```python
from build123d import *

# Parameters (mm, degrees)
ESQUISSE1_R             = 34.9
BOSS_EXTRU_1_DEPTH      = 4
ESQUISSE4_W             = 3
ESQUISSE4_H             = 15
BOSS_EXTRU_3_DEPTH      = 20
ENL_V_MAT_EXTRU_2_DEPTH = 57.306038753
CONG_1_R                = 5
ESQUISSE6_R             = 2.5
ENL_V_MAT_EXTRU_3_DEPTH = 55.995032503
BOSS_EXTRU_4_DEPTH      = 2
CONG_2_R                = 2


with BuildPart() as part:
    # Esquisse1 → Boss.-Extru.1 (new body)
    with BuildSketch(Plane.XY):
        Circle(ESQUISSE1_R)
    extrude(amount=BOSS_EXTRU_1_DEPTH)

    # Esquisse4 → Boss.-Extru.3 (add)
    with BuildSketch(Plane(origin=(0, 0, 0), x_dir=(-1, 0, 0), z_dir=(0, 0, -1))):
        with Locations((3, 0)):
            Rectangle(ESQUISSE4_W, ESQUISSE4_H)
        with Locations((-3, 0)):
            Rectangle(ESQUISSE4_W, ESQUISSE4_H)
    extrude(amount=BOSS_EXTRU_3_DEPTH)

    # Esquisse5 → Enlèv. mat.-Extru.2 (cut, through all)
    with BuildSketch(Plane(origin=(4.5, 0, 0), x_dir=(0, 0, -1), z_dir=(1, 0, 0))):
        with BuildLine():
            Line((8.44, 7.5), (20, 7.5))
            Line((20, 7.5), (20, -7.5))
            Line((20, -7.5), (8.44, -7.5))
            ThreePointArc((8.44, -7.5), (15.94, 0), (8.44, 7.5))
        make_face()
    extrude(amount=-ENL_V_MAT_EXTRU_2_DEPTH, mode=Mode.SUBTRACT)

    # Congé1
    cong_1_edges = [part.edges().sort_by_distance(p)[0] for p in [
        (-3, 7.5, 0),
        (-3, -7.5, 0),
        (-4.5, 0, 0),
        (4.5, 0, 0),
        (3, -7.5, 0),
        (3, 7.5, 0),
    ]]
    fillet(cong_1_edges, radius=CONG_1_R)

    # Esquisse6 → Enlèv. mat.-Extru.3 (cut, through all)
    with BuildSketch(Plane(origin=(4.5, 0, 0), x_dir=(0, 0, -1), z_dir=(1, 0, 0))):
        with Locations((8.44, 0)):
            Circle(ESQUISSE6_R)
    extrude(amount=-ENL_V_MAT_EXTRU_3_DEPTH, mode=Mode.SUBTRACT)

    # Esquisse2 → Boss.-Extru.4 (add)
    with BuildSketch(Plane.XY.offset(4)):
        with BuildLine():
            ThreePointArc((-11.241763565, -30.600371762), (0, 32.6), (11.241763565, -30.600371762))
            Line((11.241763565, -30.600371762), (-11.241763565, -30.600371762))
        make_face()
        with BuildLine():
            Line((-10.880199222, -28.600371762), (10.880199222, -28.600371762))
            ThreePointArc((10.880199222, -28.600371762), (0, 30.6), (-10.880199222, -28.600371762))
        make_face(mode=Mode.SUBTRACT)
    extrude(amount=BOSS_EXTRU_4_DEPTH)

    # Congé2
    cong_2_edges = [part.edges().sort_by_distance(p)[0] for p in [
        (-34.9, 0, 0),
    ]]
    fillet(cong_2_edges, radius=CONG_2_R)


solid = part.part
```
For this review, take the finished solid that the model builds, in its own axes (mm). A direction names the side the tool comes from. Round coordinates to 2 decimals unless told otherwise and drop trailing zeros. Write each loop counter-clockwise with the first axis right and the second up, starting at its lowest first coordinate (ties: lowest second). Pieces come first, ordered by that corner, then holes. Notation, with made-up numbers: (-32, 83) - (0, 83) arc R14 ccw to (0, 92) - close; hole circle Ø2 at (54.5, 70.5). An arc over 180 degrees is marked (long way). Answer as a JSON object with one key per item and string values.
1. Tool access review of faces 4 (the face through (4.5, 0, -12)), 5 (the face through (0, -30.6, 5)), 6 (the face through (0, 1, 4)), 7 (the face through (-3, 7.5, -7)), 8 (the face through (-4.5, 0, -12)): name each direction out of +Z, -Z, +X, -X, +Y, -Y from which nothing blocks a thin tool from reaching the whole face with its end or side.
Response values:
{"face 4": "-Z, +X, +Y, -Y", "face 5": "+Z, +X, -X, -Y", "face 6": "+Z", "face 7": "-Z, +X, -X, +Y", "face 8": "-Z, -X, +Y, -Y"}
2. We need section D-D on z = -14. Give the boundary of the cut face in (x, y).
Response values:
{"outline": "(-4.5, -5.03) - (-1.5, -5.03) - (-1.5, 5.03) - (-4.5, 5.03) - close; (1.5, -5.03) - (4.5, -5.03) - (4.5, 5.03) - (1.5, 5.03) - close"}
3. We need section B-B on x = 0. Give the boundary of the cut face in (y, z), then the cut area to 3 significant figures.
Response values:
{"outline": "(-34.9, 2) arc R2 ccw to (-32.9, 0) - (32.9, 0) arc R2 ccw to (34.9, 2) - (34.9, 4) - (32.6, 4) - (32.6, 6) - (30.6, 6) - (30.6, 4) - (-28.6, 4) - (-28.6, 6) - (-30.6, 6) - (-30.6, 4) - (-34.9, 4) - close", "area": "285 mm2"}
4. To check wall thickness, follow line 1 along X through (y, z) = (0, 5.1); line 2 along X through (y, z) = (-5, -8); line 3 along Y through (x, z) = (-2.95, -8.44). State the ranges of each line that lie inside material, in increasing order.
Response values:
{"line 1": "x = -32.6 to -30.6, 30.6 to 32.6", "line 2": "x = -4.5 to -1.5, 1.5 to 4.5", "line 3": "y = -7.5 to -2.5, 2.5 to 7.5"}
5. We need section A-A on z = -9.75. Give the boundary of the cut face in (x, y), then the cut area to 3 significant figures.
Response values:
{"outline": "(-4.5, -7.38) - (-1.5, -7.38) - (-1.5, -2.13) - (-4.5, -2.13) - close; (-4.5, 2.13) - (-1.5, 2.13) - (-1.5, 7.38) - (-4.5, 7.38) - close; (1.5, -7.38) - (4.5, -7.38) - (4.5, -2.13) - (1.5, -2.13) - close; (1.5, 2.13) - (4.5, 2.13) - (4.5, 7.38) - (1.5, 7.38) - close", "area": "63.1 mm2"}
6. For pin 1 Ø12 at (x, y) = (-17.5, -26) entering from -Z; pin 2 Ø5 at (y, z) = (-24, 0) entering from +X; pin 3 Ø13 at (y, z) = (4.5, -4.5) entering from +X, all flat-tipped, find the tip position at first contact; note any pin that passes through.
Response values:
{"pin 1": "stops at z = 0", "pin 2": "stops at x = 27.04", "pin 3": "stops at x = 34.79"}
7. We need section C-C on y = 0. Count the separate pieces of the cut face and the enclosed holes in it, then the cut area to 3 significant figures.
Response values:
{"separate pieces": "3", "enclosed holes": "0", "area": "362 mm2"}
8. Draft analysis for pull direction X (two halves, no side actions). For faces 1 (the face through (-1.5, -3, -8)), 2 (the face through (-3, -7.5, -7)), 3 (the face through (-1.273, 32.575, 4.986)), state which applies: +X half, -X half, draft (parallel to the pull), parting line (faces both ways), or undercut.
Response values:
{"face 1": "undercut", "face 2": "draft", "face 3": "parting line"}
